from build123d import *

# Parameters (mm, degrees)
SKETCH1_R           = 75
BOSS_EXTRUDE1_DEPTH = 5
SKETCH3_R           = 1.5
SKETCH3_W           = 40.3
SKETCH3_H           = 20
SKETCH3_W_2         = 20
SKETCH3_H_2         = 40.3
CUT_EXTRUDE1_DEPTH  = 5
SKETCH4_R           = 90
CUT_EXTRUDE2_DEPTH  = 5
SKETCH5_R           = 2.5
SKETCH5_R_2         = 10
SKETCH5_R_3         = 1.5
CUT_EXTRUDE3_DEPTH  = 5


with BuildPart() as part:
    # Sketch1 → Boss-Extrude1 (new body)
    with BuildSketch(Plane(origin=(0, 0, 0), x_dir=(1, 0, 0), z_dir=(0, 1, 0))):
        with Locations(Location((0, 0, 0), (0, 0, 270))):
            Circle(SKETCH1_R)
    extrude(amount=BOSS_EXTRUDE1_DEPTH)

    # Sketch3 → Cut-Extrude1 (cut)
    with BuildSketch(Plane(origin=(0, 5, 0), x_dir=(1, 0, 0), z_dir=(0, 1, 0))):
        with Locations(Location((-14.7, 5, 0), (0, 0, 270))):
            Circle(SKETCH3_R)
        with Locations(Location((-14.7, -5, 0), (0, 0, 270))):
            Circle(SKETCH3_R)
        with Locations(Location((-63, 5, 0), (0, 0, 270))):
            Circle(SKETCH3_R)
        with Locations(Location((-63, -5, 0), (0, 0, 270))):
            Circle(SKETCH3_R)
        with Locations(Location((-5, -14.7, 0), (0, 0, 270))):
            Circle(SKETCH3_R)
        with Locations(Location((5, -14.7, 0), (0, 0, 270))):
            Circle(SKETCH3_R)
        with Locations(Location((14.7, 5, 0), (0, 0, 270))):
            Circle(SKETCH3_R)
        with Locations(Location((14.7, -5, 0), (0, 0, 270))):
            Circle(SKETCH3_R)
        with Locations(Location((-5, 14.7, 0), (0, 0, 270))):
            Circle(SKETCH3_R)
        with Locations(Location((5, 14.7, 0), (0, 0, 270))):
            Circle(SKETCH3_R)
        with Locations(Location((-5, -63, 0), (0, 0, 270))):
            Circle(SKETCH3_R)
        with Locations(Location((5, -63, 0), (0, 0, 270))):
            Circle(SKETCH3_R)
        with Locations(Location((63, 5, 0), (0, 0, 270))):
            Circle(SKETCH3_R)
        with Locations(Location((63, -5, 0), (0, 0, 270))):
            Circle(SKETCH3_R)
        with Locations(Location((-5, 63, 0), (0, 0, 270))):
            Circle(SKETCH3_R)
        with Locations(Location((5, 63, 0), (0, 0, 270))):
            Circle(SKETCH3_R)
        with Locations((-38.85, 0)):
            Rectangle(SKETCH3_W, SKETCH3_H)
        with Locations((38.85, 0)):
            Rectangle(SKETCH3_W, SKETCH3_H)
        with Locations((0, 38.85)):
            Rectangle(SKETCH3_W_2, SKETCH3_H_2)
        with Locations((0, -38.85)):
            Rectangle(SKETCH3_W_2, SKETCH3_H_2)
    extrude(amount=-CUT_EXTRUDE1_DEPTH, mode=Mode.SUBTRACT)

    # Sketch4 → Cut-Extrude2 (cut)
    with BuildSketch(Plane(origin=(0, 5, 0), x_dir=(1, 0, 0), z_dir=(0, 1, 0))):
        with Locations((-100, 100)):
            Circle(SKETCH4_R)
        with Locations((100, 100)):
            Circle(SKETCH4_R)
        with Locations((100, -100)):
            Circle(SKETCH4_R)
        with Locations((-100, -100)):
            Circle(SKETCH4_R)
    extrude(amount=-CUT_EXTRUDE2_DEPTH, mode=Mode.SUBTRACT)

    # Sketch5 → Cut-Extrude3 (cut)
    with BuildSketch(Plane(origin=(0, 5, 0), x_dir=(1, 0, 0), z_dir=(0, 1, 0))):
        with Locations(Location((-30, 30, 0), (0, 0, 270))):
            Circle(SKETCH5_R)
        with Locations(Location((30, 30, 0), (0, 0, 270))):
            Circle(SKETCH5_R)
        with Locations(Location((30, -30, 0), (0, 0, 270))):
            Circle(SKETCH5_R)
        with Locations(Location((-30, -30, 0), (0, 0, 270))):
            Circle(SKETCH5_R)
        with Locations(Location((0, 0, 0), (0, 0, 270))):
            Circle(SKETCH5_R_2)
        with Locations(Location((-37.071067812, -22.928932188, 0), (0, 0, 270))):
            Circle(SKETCH5_R_3)
        with Locations(Location((-22.928932188, -37.071067812, 0), (0, 0, 270))):
            Circle(SKETCH5_R_3)
        with Locations(Location((22.928932188, -37.071067812, 0), (0, 0, 270))):
            Circle(SKETCH5_R_3)
        with Locations(Location((37.071067812, -22.928932188, 0), (0, 0, 270))):
            Circle(SKETCH5_R_3)
        with Locations(Location((37.071067812, 22.928932188, 0), (0, 0, 270))):
            Circle(SKETCH5_R_3)
        with Locations(Location((22.928932188, 37.071067812, 0), (0, 0, 270))):
            Circle(SKETCH5_R_3)
        with Locations(Location((-22.928932188, 37.071067812, 0), (0, 0, 270))):
            Circle(SKETCH5_R_3)
        with Locations(Location((-37.071067812, 22.928932188, 0), (0, 0, 270))):
            Circle(SKETCH5_R_3)
    extrude(amount=-CUT_EXTRUDE3_DEPTH, mode=Mode.SUBTRACT)


solid = part.part
Geometry check sheet. Reference: the model listing, model coordinates, mm. A direction names the side the tool comes from. Give positions to 0.01 mm unless a question says otherwise; leave off trailing zeros. Loops run counter-clockwise (first coordinate to the right, second up) from the corner with the lowest first, then second, coordinate; pieces in that order, holes last.
(1) Section check C-C on y = 2. Count the separate pieces of the cut face and the enclosed holes in it, then the cut area to 3 significant figures.
From the geometry:
separate pieces: 1
enclosed holes: 33
area: 8,490 mm2
(2) Set-up check for faces 1 (the flat face through (0, 3, -18.7)), 2 (the cylindrical face through (-36.797, 2.535, -35.926)): record each of +Z, -Z, +X, -X, +Y, -Y from which the full face is reachable in a straight line by a thin tool's end or side.
From the geometry:
face 1: +Y, -Y
face 2: -Z, -X, +Y, -Y
(3) Section check B-B on x = -42. Record the cut outline in (y, z), then the cut area to 3 significant figures.
From the geometry:
outline: (0, -31.18) - (5, -31.18) - (5, -10) - (0, -10) - close; (0, 10) - (5, 10) - (5, 31.18) - (0, 31.18) - close
area: 212 mm2
(4) Section check A-A on z = -52. Record the cut outline in (x, y).
From the geometry:
outline: (-23.87, 0) - (-10, 0) - (-10, 5) - (-23.87, 5) - close; (10, 0) - (23.87, 0) - (23.87, 5) - (10, 5) - close
(5) Release check for a two-part mould opening along Z. For faces 3 (the flat face through (-16, 5, -1)), 4 (the cylindrical face through (-27.52, 2.54, 29.67)), 5 (the cylindrical face through (0, 2, 75)), 6 (the cylindrical face through (31.69, 2.54, -31.84)) record: released by +Z, released by -Z, zero draft, split by the parting line, or undercut.
From the geometry:
face 3: zero draft
face 4: undercut
face 5: released by +Z
face 6: undercut
(6) Thickness scan on L1, parallel to Z at x = -0.5, y = 3.7; L2, parallel to X at y = 0.7, z = -2.5; L3, parallel to X at y = 1.2, z = 63. Record the ranges inside material, lowest first.
From the geometry:
L1: z = -75 to -59, -18.7 to -9.99, 9.99 to 18.7, 59 to 75
L2: x = -74.96 to -59, -18.7 to -9.68, 9.68 to 18.7, 59 to 74.96
L3: x = -17.96 to -6.5, -3.5 to 3.5, 6.5 to 17.96
(7) Depth check by flat-ended pin: pin 1 Ø1.5 at (x, y) = (-9, 2) entering from -Z; pin 2 Ø6 at (x, z) = (-30, 30) entering from -Y; pin 3 Ø2 at (x, y) = (-18.5, 4) entering from -Z; pin 4 Ø2.5 at (y, z) = (2.5, 32) entering from +X. Enter the tip coordinate at first touch or a pass-through.
From the geometry:
pin 1: stops at z = -74.54
pin 2: stops at y = 0
pin 3: stops at z = -64.03
pin 4: stops at x = 42.52
